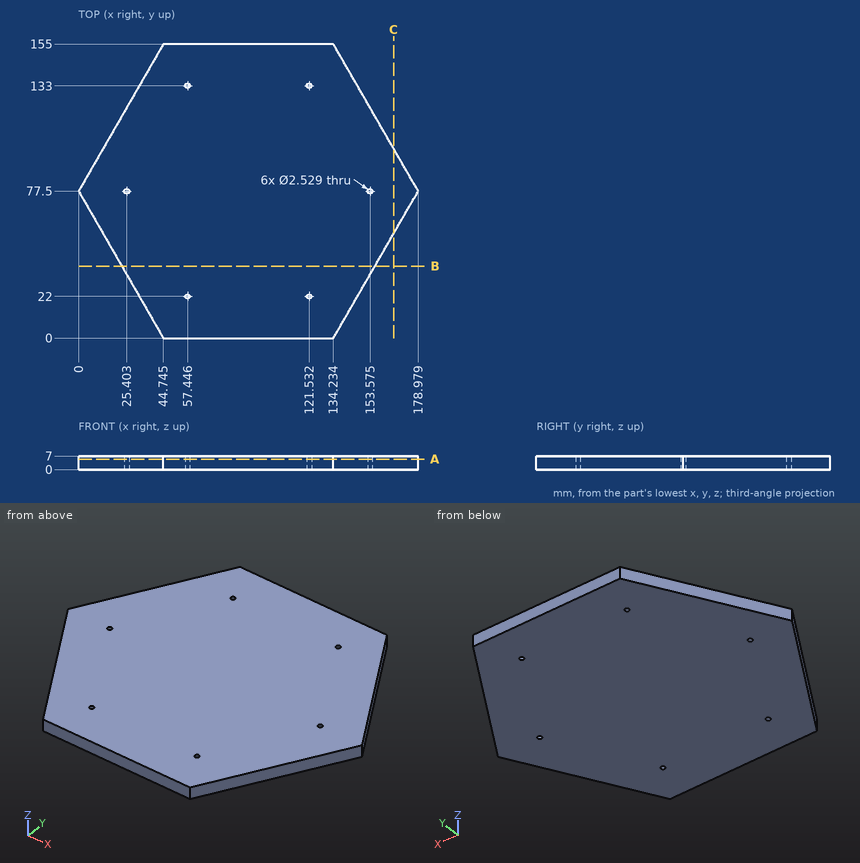
Could you check a few things on this drawing? It's one solid part, dimensions in mm from its lowest x, y, z. Coordinates: 2 decimals unless noted, no trailing zeros. Write each loop counter-clockwise with the first axis right and the second up, starting at its lowest first coordinate (ties: lowest second). Pieces come first, ordered by that corner, then holes.
1) If we section it at B-B (y = 38): List the corners of the cut face in (x, z) for me (1 decimal).
Filled in:
outline: (22.8, 0) - (156.2, 0) - (156.2, 7) - (22.8, 7) - close
2) If we section it at C-C (x = 166): List the corners of the cut face in (y, z) for me, plus the area to 3 significant figures.
Filled in:
outline: (55.02, 0) - (99.98, 0) - (99.98, 7) - (55.02, 7) - close
area: 315 mm2
3) I'm going to push flat-ended pins straight in: pin 1 (1.5 mm diameter, centred on y = 61, z = 4.5, fed in from +X) (1 decimal); pin 2 (2 mm diameter, centred on y = 120, z = 5.5, fed in from -X); pin 3 (2 mm diameter, centred on y = 49.5, z = 2.5, fed in from +X). Where does each tip first touch, or does it pass through?
Filled in:
pin 1: stops at x = 169.9
pin 2: stops at x = 23.96
pin 3: stops at x = 163.39
4) If I drill on line 1 (X direction, y = 133, z = 3.25) (1 decimal); line 2 (Y direction, x = 153, z = 3.25) (1 decimal); line 3 (X direction, y = 97, z = 2.25), over which ranges is the centre line in solid material (lowest first)?
Filled in:
line 1: x = 32 to 56.2, 58.7 to 120.3, 122.8 to 146.9
line 2: y = 32.5 to 76.4, 78.6 to 122.5
line 3: x = 11.26 to 167.72
5) If we section it at A-A (z = 5.5): List the corners of the cut face in (x, y) for me (1 decimal).
Filled in:
outline: (0, 77.5) - (44.7, 0) - (134.2, 0) - (179, 77.5) - (134.2, 155) - (44.7, 155) - close; hole circle Ø2.5 at (25.4, 77.5); hole circle Ø2.5 at (57.4, 22); hole circle Ø2.5 at (57.4, 133); hole circle Ø2.5 at (121.5, 22); hole circle Ø2.5 at (121.5, 133); hole circle Ø2.5 at (153.6, 77.5)
